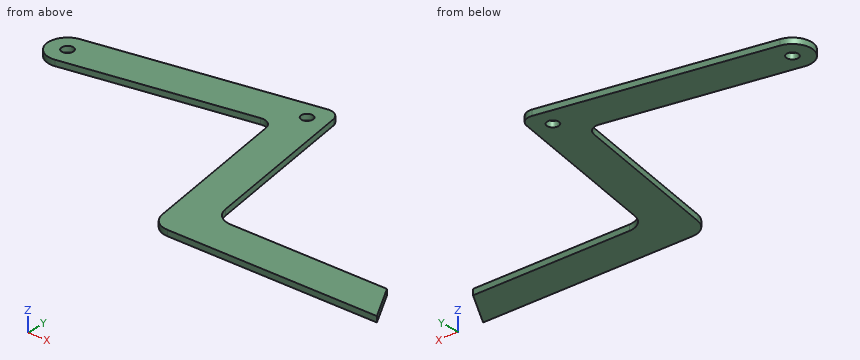
from build123d import *

# Parameters (mm, degrees)
SKETCH1_R           = 1.5
BOSS_EXTRUDE1_DEPTH = 0.75


with BuildPart() as part:
    # Sketch1 → Boss-Extrude1 (new body, symmetric)
    with BuildSketch(Plane.XY):
        with BuildLine():
            Line((4.195498156, 0), (60, 0))
            Line((60, 0), (54.226497308, 10))
            Line((54.226497308, 10), (12.586494468, 10))
            ThreePointArc((12.586494468, 10), (9.372556419, 11.169777784), (7.662455703, 14.131759112))
            Line((7.662455703, 14.131759112), (0.095591809, 57.045576741))
            ThreePointArc((0.095591809, 57.045576741), (-1.138102141, 58.982088341), (-3.379775983, 59.479055467))
            Line((-3.379775983, 59.479055467), (-60.868240888, 49.342288025))
            ThreePointArc((-60.868240888, 49.342288025), (-64.924038765, 43.550008371), (-59.131759112, 39.494210494))
            Line((-59.131759112, 39.494210494), (-11.491371736, 47.89449616))
            ThreePointArc((-11.491371736, 47.89449616), (-9.249697894, 47.397529034), (-8.016003944, 45.461017434))
            Line((-8.016003944, 45.461017434), (-0.728540609, 4.131759112))
            ThreePointArc((-0.728540609, 4.131759112), (0.981560107, 1.169777784), (4.195498156, 0))
        make_face()
        with Locations((-60, 44.41824926)):
            Circle(SKETCH1_R, mode=Mode.SUBTRACT)
        with Locations((-4.4811506, 54.207720347)):
            Circle(SKETCH1_R, mode=Mode.SUBTRACT)
    extrude(amount=BOSS_EXTRUDE1_DEPTH, both=True)


solid = part.part
Source: CAD feature listing. Evaluate the final solid. Frame: model axes, mm. Round coordinates to 2 decimals unless told otherwise and drop trailing zeros. Loops run counter-clockwise (first coordinate to the right, second up) from the corner with the lowest first, then second, coordinate; pieces in that order, holes last. Notation, with made-up numbers: M -34,54.5 L -11,54.5 A15 ccw -11,82.5 Z; hole C -26.75,2.25 d1. An arc over 180 degrees is marked long. Answer as CSV lines item,"result".
Q1. Cut plane B-B (z = -0.1). Return the cut outline in (x, y), plus the area to 3 significant figures.
Verdict:
outline,"M -60.87,49.34 A5 ccw -59.13,39.49 L -11.49,47.89 A3 cw -8.02,45.46 L -0.73,4.13 A5 ccw 4.2,0 L 60,0 L 54.23,10 L 12.59,10 A5 cw 7.66,14.13 L 0.1,57.05 A3 ccw -3.38,59.48 Z; hole C -60,44.42 d3; hole C -4.48,54.21 d3"
area,"1,620 mm^2"
Q2. Line query: line 1 along Y through (x, z) = (50, 0.6); line 2 along X through (y, z) = (30.5, 0.1); line 3 along Y through (x, z) = (-41.5, 0.5). Output: solid intervals per line, ascending.
Verdict:
line 1,"y = 0 to 10"
line 2,"x = -5.38 to 4.78"
line 3,"y = 42.6 to 52.76"
Q3. Cut plane C-C (x = 25). Return the cut outline in (y, z).
Verdict:
outline,"M 0,-0.75 L 10,-0.75 L 10,0.75 L 0,0.75 Z"
Q4. Cut plane A-A (y = 41.5). Return the cut outline in (x, z), plus the area to 3 significant figures.
Verdict:
outline,"M -64.06,-0.75 L -47.76,-0.75 L -47.76,0.75 L -64.06,0.75 Z; M -7.32,-0.75 L 2.84,-0.75 L 2.84,0.75 L -7.32,0.75 Z"
area,"39.7 mm^2"
Q5. Cut plane D-D (y = 7). Return the cut outline in (x, z), plus the area to 3 significant figures.
Verdict:
outline,"M -1.23,-0.75 L 55.96,-0.75 L 55.96,0.75 L -1.23,0.75 Z"
area,"85.8 mm^2"
